CAD build for the part. Positions are in the model's coordinates, mm. A direction names the side the tool comes from. Give positions to 0.01 mm unless a question says otherwise; leave off trailing zeros. Loops run counter-clockwise (first coordinate to the right, second up) from the corner with the lowest first, then second, coordinate; pieces in that order, holes last.
```python
from build123d import *

# Parameters (mm, degrees)
F0_W     = 36.8556268513
F0_H     = 23.1989044696
F1_DEPTH = 30.48
F3_DEPTH = 40.132
F4_DEPTH = 52.578
F5_DEPTH = 77.978
F6_R     = 1.0180140376
F7_DEPTH = 4.1148
F8_R     = 1.6548537216
F9_DEPTH = 43.8912


with BuildPart() as f1:
    # F0 (on Front) → F1 (new body)
    with BuildSketch(Plane.XZ):
        with Locations((-18.4278134257, 11.5994522348)):
            Rectangle(F0_W, F0_H)
    extrude(amount=F1_DEPTH)

    # F2 (on face) → F3 (join)
    with BuildSketch(Plane.XZ.offset(30.48)):
        with BuildLine():
            ThreePointArc((-6.3564511947, 23.1989044696), (-18.7693366315, 17.1609803007), (-31.1822220683, 23.1989044696))
            Line((-31.1822220683, 23.1989044696), (-33.6186587811, 23.1989044696))
            ThreePointArc((-33.6186587811, 23.1989044696), (-18.3155420236, 13.3691620993), (-3.0124252662, 23.1989044696))
            Line((-3.0124252662, 23.1989044696), (-6.3564511947, 23.1989044696))
        make_face()
    extrude(amount=-F3_DEPTH)

    # F4 (add): a face of the model
    f4_faces = [f1.faces().sort_by_distance(p)[0] for p in [
        (-18.3155420236, 9.652, 13.690622107),
    ]]
    extrude(f4_faces, amount=-F4_DEPTH)

    # F5 (cut): a face of the model
    f5_faces = [f1.faces().sort_by_distance(p)[0] for p in [
        (-18.7693366315, -30.48, 20.7391498163),
    ]]
    extrude(f5_faces, amount=-F5_DEPTH, mode=Mode.SUBTRACT)

    # F6 (on face) → F7 (cut)
    with BuildSketch(Plane.XY.offset(23.1989044696)):
        with Locations((-34.3416407704, -15.24)):
            Circle(F6_R)
    extrude(amount=-F7_DEPTH, mode=Mode.SUBTRACT)

    # F8 (on face) → F9 (cut)
    with BuildSketch(Plane.XY.offset(23.1989044696)):
        with Locations((-2.1695073228, -15.4512235895)):
            Circle(F8_R)
    extrude(amount=-F9_DEPTH, mode=Mode.SUBTRACT)


solid = f1.part
```
1. Tool access for faces 1 (the face through (-19, -42.926, 16)), 2 (the face through (-18.58, -36.62, 13.37)), 3 (the face through (-35.36, -15.2, 21.17)): list every direction of +Z, -Z, +X, -X, +Y, -Y with a clear straight run to the whole face (end or side of a thin tool).
Responses:
face 1: +Z, -Z, +X, -X, -Y
face 2: -Z, -Y
face 3: +Z
2. Drop flat-ended pins along their axis: pin 1 (10 mm diameter, centred on x = -27, z = 20, fed in from -Y); pin 2 (1.8 mm diameter, centred on x = -34.34, y = -15.24, fed in from +Z); pin 3 (1 mm diameter, centred on x = -27.5, y = -7, fed in from +Z); pin 4 (8 mm diameter, centred on x = -16.5, y = -2, fed in from +Z). Give the stop position or say it passes through.
Responses:
pin 1: stops at y = -42.93
pin 2: stops at z = 19.08
pin 3: stops at z = 20.14
pin 4: stops at z = 18.46
3. Saw through at D-D, the plane y = 3. List the corners of the cut face in (x, z).
Responses:
outline: (-33.62, 23.2) arc R16.83 ccw to (-3.01, 23.2) - (-6.36, 23.2) arc R15.78 cw to (-31.18, 23.2) - close
4. Probe line 1 along Y through (x, z) = (-2, 18.25); line 2 along Y through (x, z) = (-30.5, 7); line 3 along X through (y, z) = (3.5, 20.75). List the from-to ranges inside material, lowest first.
Responses:
line 1: y = -30.48 to -17.1, -13.81 to 0
line 2: y = -30.48 to 0
line 3: x = -32.24 to -28.79, -8.75 to -4.39
5. Saw through at A-A, the plane y = -28. List the corners of the cut face in (x, z).
Responses:
outline: (-36.86, 0) - (0, 0) - (0, 23.2) - (-6.36, 23.2) arc R15.78 cw to (-31.18, 23.2) - (-36.86, 23.2) - close
6. Saw through at C-C, the plane x = -18.5. List the corners of the cut face in (y, z).
Responses:
outline: (-42.93, 13.37) - (-30.48, 13.37) - (-30.48, 0) - (0, 0) - (0, 13.37) - (9.65, 13.37) - (9.65, 17.16) - (-42.93, 17.16) - close
7. Saw through at B-B, the plane x = -30.5. List the corners of the cut face in (y, z).
Responses:
outline: (-42.93, 18.59) - (-30.48, 18.59) - (-30.48, 0) - (0, 0) - (0, 18.59) - (9.65, 18.59) - (9.65, 22.39) - (-42.93, 22.39) - close
8. Pull direction Y, two halves, no side cores. Call faces 4 (the face through (-18.58, 4.76, 13.37)), 5 (the face through (-2.38, -13.81, 11.76)), 6 (the face through (-19, 9.652, 16)): released by +Y, released by -Y, zero draft, split by the parting line, or undercut.
Responses:
face 4: zero draft
face 5: undercut
face 6: released by +Y
